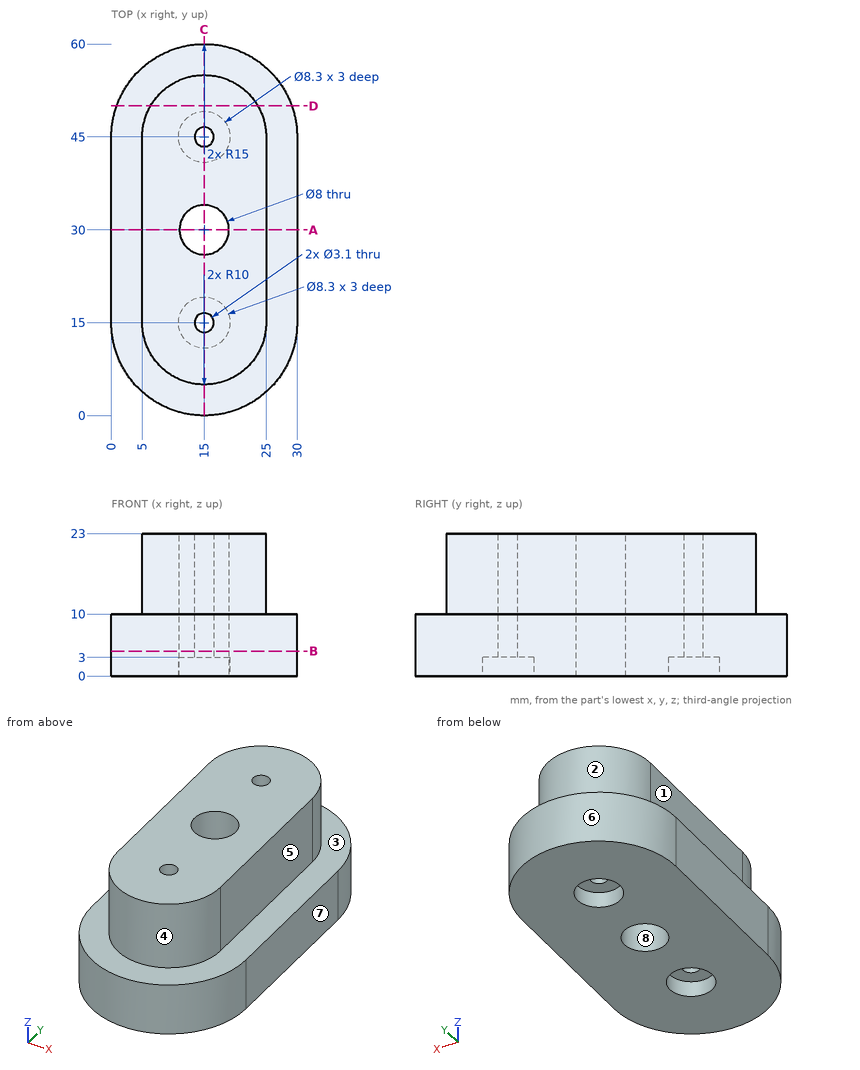
Can you work these out from the drawing? Everything is in mm from the part's minimum corner. A direction names the side the tool comes from. Coordinates: 2 decimals unless noted, no trailing zeros. Loops run counter-clockwise (first coordinate to the right, second up) from the corner with the lowest first, then second, coordinate; pieces in that order, holes last.
1) Will these pins go through, and if not, where does the flat tip stop? pin 1 Ø4 at (y, z) = (48.5, 20.5) entering from +X; pin 2 Ø10.5 at (y, z) = (33.5, 16) entering from -X; pin 3 Ø2 at (y, z) = (7.5, 10) entering from +X; pin 4 Ø6.5 at (x, y) = (15, 30) entering from +Z.
Reported:
pin 1: stops at x = 24.89
pin 2: stops at x = 5
pin 3: stops at x = 28.52
pin 4: passes through
2) Imagine slicing it at D-D (y = 50). List the corners of the cut face in (x, z) for me.
Reported:
outline: (0.86, 0) - (29.14, 0) - (29.14, 10) - (23.66, 10) - (23.66, 23) - (6.34, 23) - (6.34, 10) - (0.86, 10) - close
3) Thinking about a two-plate mould opening in X: for the marked faces 6, 7 and 8, which applies, released by +X, released by -X, zero draft, split by the parting line, or undercut?
Reported:
face 6: split by the parting line
face 7: released by +X
face 8: undercut
4) Imagine slicing it at B-B (z = 4). List the corners of the cut face in (x, y) for me.
Reported:
outline: (0, 15) arc R15 ccw to (30, 15) - (30, 45) arc R15 ccw to (0, 45) - close; hole circle Ø8 at (15, 30); hole circle Ø3.1 at (15, 15); hole circle Ø3.1 at (15, 45)
5) Please list where these lines run through material, in increasing order: line 1 along Y through (x, z) = (15, 0.9); line 2 along Y through (x, z) = (15, 8); line 3 along Z through (x, y) = (10.5, 57.5).
Reported:
line 1: y = 0 to 10.85, 19.15 to 26, 34 to 40.85, 49.15 to 60
line 2: y = 0 to 13.45, 16.55 to 26, 34 to 43.45, 46.55 to 60
line 3: z = 0 to 10
6) Which directions (+Z, -Z, +X, -X, +Y, -Y) give clear straight access to the entire face, cutting with the end or side of a thin tool? Please do the marked faces 1, 2, 3, 4 and 5.
Reported:
face 1: +Z, -X, +Y, -Y
face 2: +Z, +Y
face 3: +Z
face 4: +Z, -Y
face 5: +Z, +X, +Y, -Y
7) Imagine slicing it at A-A (y = 30). List the corners of the cut face in (x, z) for me.
Reported:
outline: (0, 0) - (11, 0) - (11, 23) - (5, 23) - (5, 10) - (0, 10) - close; (19, 0) - (30, 0) - (30, 10) - (25, 10) - (25, 23) - (19, 23) - close
8) Imagine slicing it at C-C (x = 15). List the corners of the cut face in (y, z) for me, and give its area (3 significant figures).
Reported:
outline: (0, 0) - (10.85, 0) - (10.85, 3) - (13.45, 3) - (13.45, 23) - (5, 23) - (5, 10) - (0, 10) - close; (16.55, 3) - (19.15, 3) - (19.15, 0) - (26, 0) - (26, 23) - (16.55, 23) - close; (34, 0) - (40.85, 0) - (40.85, 3) - (43.45, 3) - (43.45, 23) - (34, 23) - close; (46.55, 3) - (49.15, 3) - (49.15, 0) - (60, 0) - (60, 10) - (55, 10) - (55, 23) - (46.55, 23) - close
area: 892 mm2
